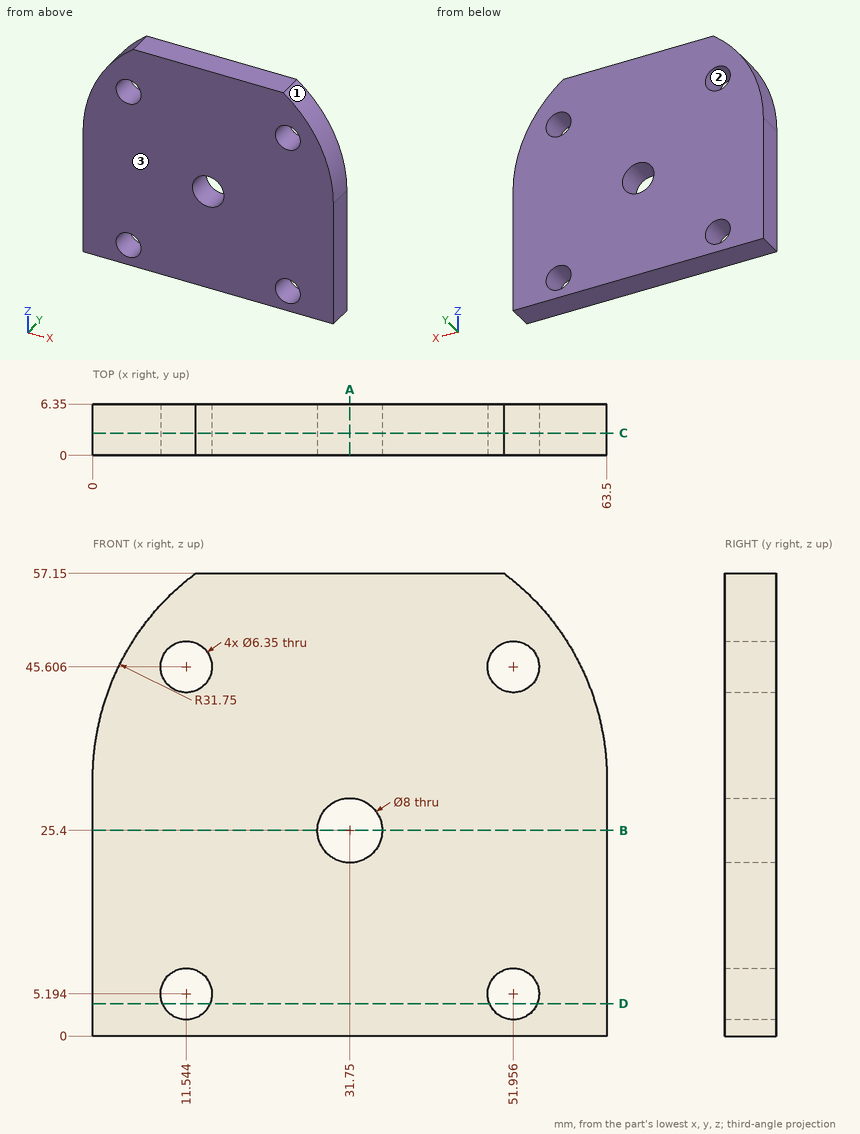
Here's the drawing with two shaded views (mm, measured from the low corner). I have some questions. Give positions to 0.01 mm unless a question says otherwise; leave off trailing zeros. Write each loop counter-clockwise with the first axis right and the second up, starting at its lowest first coordinate (ties: lowest second). Pieces come first, ordered by that corner, then holes. Notation, with made-up numbers: (26.25, 87) -> (62.25, 87) arc R22 ccw to (62.25, 108) -> close; hole circle Ø6 at (-23, 65). An arc over 180 degrees is marked (long way). Answer as a JSON object with one key per item and string values. Group by question number.
Item 1: Suppose I cut it at B-B (z = 25.4). Please give me the cut outline in (x, y).
Item 2: I'm going to push a flat-ended pin straight in: P1, Ø1, axis at y = 1, z = 35.5, coming from the -X side. Where does the tip first touch, or does it pass through?
Item 3: We'd pull the mould along X, two halves only. Please class the marked faces 1, 2 and 3: +X half, -X half, draft (parallel to the pull), parting line (faces both ways), or undercut.
Item 4: Suppose I cut it at A-A (x = 31.75). Please give me the cut outline in (y, z), plus the area to 3 significant figures.
Item 5: Suppose I cut it at D-D (z = 4). Please give me the cut outline in (x, y).
Item 6: Suppose I cut it at C-C (y = 2.75). State how many separate pieces and enclosed holes the cut face has, plus the area to 3 significant figures.
Item 7: Please list where these lines run through material, in increasing order: line 1 (X direction, y = 4, z = 25.4); line 2 (X direction, y = 4.25, z = 4) (1 decimal); line 3 (Z direction, x = 53, y = 0.75) (1 decimal). Write a range as [from, to].
Findings:
{
 "1": {"outline": "(0, 0) -> (27.75, 0) -> (27.75, 6.35) -> (0, 6.35) -> close; (35.75, 0) -> (63.5, 0) -> (63.5, 6.35) -> (35.75, 6.35) -> close"},
 "2": {"P1": "stops at x = 0.17"},
 "3": {"face 1": "+X half", "face 2": "undercut", "face 3": "draft"},
 "4": {"outline": "(0, 0) -> (6.35, 0) -> (6.35, 21.4) -> (0, 21.4) -> close; (0, 29.4) -> (6.35, 29.4) -> (6.35, 57.15) -> (0, 57.15) -> close", "area": "312 mm²"},
 "5": {"outline": "(0, 0) -> (8.6, 0) -> (8.6, 6.35) -> (0, 6.35) -> close; (14.49, 0) -> (49.01, 0) -> (49.01, 6.35) -> (14.49, 6.35) -> close; (54.9, 0) -> (63.5, 0) -> (63.5, 6.35) -> (54.9, 6.35) -> close"},
 "6": {"separate pieces": "1", "enclosed holes": "5", "area": "3,260 mm²"},
 "7": {"line 1": "x = [0, 27.75], [35.75, 63.5]", "line 2": "x = [0, 8.6], [14.5, 49], [54.9, 63.5]", "line 3": "z = [0, 2.2], [8.2, 42.6], [48.6, 55.3]"}
}
